Verification items for the finished model (mm, model axes). A direction names the side the tool comes from. Coordinates: 2 decimals unless noted, no trailing zeros. Order: outer loops, then holes, each group sorted by start corner. A loop starts at its lowest first (then second) coordinate and runs counter-clockwise, first axis right, second up.
Q1. Cross-section at D-D, the plane x = 17. Record the boundary of the cut face in (y, z), and give its area (3 significant figures).
Q2. Thickness scan on line 1 (Z direction, x = -20.5, y = -12); line 2 (Y direction, x = 0, z = 26); line 3 (X direction, y = 11, z = 18.5). Record the ranges inside material, lowest first.
Q3. Depth check by flat-ended pin: P1, Ø8, axis at x = 8.5, y = 2, coming from the -Z side; P2, Ø5, axis at x = 18.5, z = 15, coming from the +Y side; P3, Ø10, axis at y = 9, z = 13, coming from the +X side; P4, Ø12, axis at x = -18, z = 17.5, coming from the +Y side. Enter the tip coordinate at first touch or a pass-through.
Q4. Cross-section at A-A, the plane x = 0. Record the boundary of the cut face in (y, z).
Q5. Draft check along Y on faces 1 (the flat face through (1, -11, 0)), 2 (the flat face through (0, 15.549, 14)), 3 (the cylindrical face through (18.258, -12.329, 1.37)). Enter one of: pulls with the +Y half, pulls with the -Y half, needs draft (parallel to the pull), parting line crosses it, or undercut.
Q6. Cross-section at B-B, the plane z = 3.5. Record the boundary of the cut face in (x, y).
Q7. Set-up check for faces 4 (the cylindrical face through (11.835, 3.727, 15.227)), 5 (the flat face through (20, -9.199, 14)), 6 (the flat face through (0, -15.549, 14)), 7 (the flat face through (-5.7, -11.4, 30.886)), 8 (the flat face through (-15.549, 1, 14)): record each of +Z, -Z, +X, -X, +Y, -Y from which the full face is reachable in a straight line by a thin tool's end or side.
from build123d import *

# Parameters (mm, degrees)
F0_R     = 2.15265
F0_R_2   = 12.4079
F1_DEPTH = 30.8864
F2_R     = 2.15265
F2_R_2   = 12.4079
F2_R_3   = 10.8204
F3_DEPTH = 4.0386
F4_R     = 2.15265
F5_DEPTH = 6.35
F6_R     = 3.96875


with BuildPart() as f1:
    # F0 (on Top) → F1 (new body)
    with BuildSketch(Plane.XY):
        Polygon((15.5487902681, 15.5487902681), (-15.5487902681, 15.5487902681), (-15.5487902681, -9.1987902681), (-25.0737902681, -9.1987902681), (-25.0737902681, -15.5487902681), (25.0737902681, -15.5487902681), (25.0737902681, -9.1987902681), (15.5487902681, -9.1987902681), align=None)
        with Locations((-11.5800402681, -11.5800402681)):
            Circle(F0_R, mode=Mode.SUBTRACT)
        with Locations((11.5800402681, -11.5800402681)):
            Circle(F0_R, mode=Mode.SUBTRACT)
        with Locations((-11.5800402681, 11.5800402681)):
            Circle(F0_R, mode=Mode.SUBTRACT)
        Circle(F0_R_2, mode=Mode.SUBTRACT)
        with Locations((11.5800402681, 11.5800402681)):
            Circle(F0_R, mode=Mode.SUBTRACT)
    extrude(amount=F1_DEPTH)

    # F2 (on face) → F3 (join)
    with BuildSketch(Plane(origin=(0, 0, 0), x_dir=(1, 0, 0), z_dir=(0, 0, -1))):
        Polygon((-15.5487902681, -15.5487902681), (15.5487902681, -15.5487902681), (15.5487902681, 9.1987902681), (25.0737902681, 9.1987902681), (25.0737902681, 15.5487902681), (-25.0737902681, 15.5487902681), (-25.0737902681, 9.1987902681), (-15.5487902681, 9.1987902681), align=None)
        with Locations((-11.5800402681, -11.5800402681)):
            Circle(F2_R, mode=Mode.SUBTRACT)
        with Locations((11.5800402681, -11.5800402681)):
            Circle(F2_R, mode=Mode.SUBTRACT)
        with Locations((-11.5800402681, 11.5800402681)):
            Circle(F2_R, mode=Mode.SUBTRACT)
        Circle(F2_R_2, mode=Mode.SUBTRACT)
        with Locations((11.5800402681, 11.5800402681)):
            Circle(F2_R, mode=Mode.SUBTRACT)
        Circle(F2_R_2)
        Circle(F2_R_3, mode=Mode.SUBTRACT)
    extrude(amount=F3_DEPTH)

    # F4 (on face) → F5 (cut, through all)
    with BuildSketch(Plane(origin=(0, -9.1987902681, 0), x_dir=(-1, 0, 0), z_dir=(0, 1, 0))):
        with Locations((-20.3112902681, 0.7239)):
            Circle(F4_R)
        with Locations((-20.3112902681, 26.1239)):
            Circle(F4_R)
        with Locations((20.3112902681, 26.1239)):
            Circle(F4_R)
        with Locations((20.3112902681, 0.7239)):
            Circle(F4_R)
    extrude(amount=-F5_DEPTH, mode=Mode.SUBTRACT)

    # F6
    f6_edges = [f1.edges().sort_by_distance(p)[0] for p in [
        (-15.54879, 15.54879, 13.4239),
        (15.54879, 15.54879, 13.4239),
    ]]
    fillet(f6_edges, radius=F6_R)


solid = f1.part
Check values:
1. outline: (-15.55, -4.04) - (-9.2, -4.04) - (-9.2, 30.89) - (-15.55, 30.89) - close
1. area: 222 mm2
2. line 1: z = -4.04 to -1.42, 2.87 to 23.98, 28.27 to 30.89
2. line 2: y = -15.55 to -12.41, 12.41 to 15.55
2. line 3: x = -15.55 to -13.65, -9.51 to -5.74, 5.74 to 9.51, 13.65 to 15.55
3. P1: stops at z = -4.04
3. P2: stops at y = -9.2
3. P3: stops at x = 15.55
3. P4: stops at y = 15.53
4. outline: (-15.55, -4.04) - (-10.82, -4.04) - (-10.82, 0) - (-12.41, 0) - (-12.41, 30.89) - (-15.55, 30.89) - close; (10.82, -4.04) - (15.55, -4.04) - (15.55, 30.89) - (12.41, 30.89) - (12.41, 0) - (10.82, 0) - close
5. face 1: undercut
5. face 2: pulls with the +Y half
5. face 3: needs draft
6. outline: (-25.07, -15.55) - (25.07, -15.55) - (25.07, -9.2) - (15.55, -9.2) - (15.55, 11.58) arc R3.97 ccw to (11.58, 15.55) - (-11.58, 15.55) arc R3.97 ccw to (-15.55, 11.58) - (-15.55, -9.2) - (-25.07, -9.2) - close; hole circle Ø4.31 at (-11.58, -11.58); hole circle Ø4.31 at (-11.58, 11.58); hole circle Ø24.82 at (0, 0); hole circle Ø4.31 at (11.58, -11.58); hole circle Ø4.31 at (11.58, 11.58)
7. face 4: +Z
7. face 5: +Z, -Z, +X, +Y
7. face 6: +Z, -Z, +X, -X, -Y
7. face 7: +Z, +X, -X, +Y, -Y
7. face 8: +Z, -Z, -X, +Y
